Input: part model. Units: mm. Frame: model coordinates. Face numbers are marked on the shaded views. A direction names the side the tool comes from. Coordinates: 2 decimals unless noted, no trailing zeros. Order: outer loops, then holes, each group sorted by start corner. A loop starts at its lowest first (then second) coordinate and runs counter-clockwise, first axis right, second up. Notation, with made-up numbers: (80.5, 39) -> (114.5, 39) arc R14 cw to (114.5, 59) -> close; hole circle Ø5 at (47.25, -27.5). An arc over 180 degrees is marked (long way). Use CSV: the item, a comma, the result in double quotes. Start each with the question number.
```python
from build123d import *

# Parameters (mm, degrees)
SKETCH1_W           = 197.4
SKETCH1_H           = 115
BOSS_EXTRUDE1_DEPTH = 9
BOSS_EXTRUDE2_DEPTH = 10
CUT_EXTRUDE1_DEPTH  = 9
CUT_EXTRUDE2_DEPTH  = 6
CUT_EXTRUDE3_DEPTH  = 2.5


with BuildPart() as part:
    # Sketch1 → Boss-Extrude1 (new body)
    with BuildSketch(Plane.XY):
        with Locations((0, 19.485033023)):
            Rectangle(SKETCH1_W, SKETCH1_H)
    extrude(amount=BOSS_EXTRUDE1_DEPTH)

    # Sketch2 → Boss-Extrude2 (add)
    with BuildSketch(Plane(origin=(0, 76.985033023, 0), x_dir=(1, 0, 0), z_dir=(0, 1, 0))):
        Polygon((-88.7, 10), (88.7, 10), (98.7, 0), (-98.7, 0), align=None)
    extrude(amount=-BOSS_EXTRUDE2_DEPTH)

    # Sketch3 → Cut-Extrude1 (cut)
    with BuildSketch(Plane.XY.offset(9)):
        with BuildLine():
            Line((-80.7, 64.985033023), (-40.7, 64.985033023))
            ThreePointArc((-40.7, 64.985033023), (-36.457359313, 63.22767371), (-34.7, 58.985033023))
            Line((-34.7, 58.985033023), (-34.7, -20.014966977))
            ThreePointArc((-34.7, -20.014966977), (-36.457359313, -24.257607664), (-40.7, -26.014966977))
            Line((-40.7, -26.014966977), (-80.7, -26.014966977))
            ThreePointArc((-80.7, -26.014966977), (-84.942640687, -24.257607664), (-86.7, -20.014966977))
            Line((-86.7, -20.014966977), (-86.7, 58.985033023))
            ThreePointArc((-86.7, 58.985033023), (-84.942640687, 63.22767371), (-80.7, 64.985033023))
        make_face()
    cut_extrude1 = extrude(amount=-CUT_EXTRUDE1_DEPTH, mode=Mode.SUBTRACT)

    # Sketch4 → Cut-Extrude2 (cut)
    with BuildSketch(Plane.XY.offset(9)):
        with BuildLine():
            Line((-94.7, 58.985033023), (-94.7, -20.014966977))
            ThreePointArc((-94.7, -20.014966977), (-90.599494937, -29.914461914), (-80.7, -34.014966977))
            Line((-80.7, -34.014966977), (-40.7, -34.014966977))
            ThreePointArc((-40.7, -34.014966977), (-30.800505063, -29.914461914), (-26.7, -20.014966977))
            Line((-26.7, -20.014966977), (-26.7, 58.985033023))
            ThreePointArc((-26.7, 58.985033023), (-30.800505063, 68.88452796), (-40.7, 72.985033023))
            Line((-40.7, 72.985033023), (-80.7, 72.985033023))
            ThreePointArc((-80.7, 72.985033023), (-90.599494937, 68.88452796), (-94.7, 58.985033023))
        make_face()
    cut_extrude2 = extrude(amount=-CUT_EXTRUDE2_DEPTH, mode=Mode.SUBTRACT)

    # Mirror1: Cut-Extrude1, Cut-Extrude2 across plane
    add(cut_extrude1.mirror(Plane(origin=(0, 0, 0), x_dir=(0, 0, 1), z_dir=(1, 0, 0))), mode=Mode.SUBTRACT)
    add(cut_extrude2.mirror(Plane(origin=(0, 0, 0), x_dir=(0, 0, 1), z_dir=(1, 0, 0))), mode=Mode.SUBTRACT)

    # Sketch5 → Cut-Extrude3 (cut)
    with BuildSketch(Plane(origin=(0, 76.985033023, 0), x_dir=(1, 0, 0), z_dir=(0, 1, 0))):
        with BuildLine():
            Line((-88.7, 5), (88.7, 5))
            ThreePointArc((88.7, 5), (90.613417162, 5.380602337), (92.235533906, 6.464466094))
            Line((92.235533906, 6.464466094), (98.599494937, 0.100505063))
            ThreePointArc((98.599494937, 0.100505063), (94.057568053, -2.934313455), (88.7, -4))
            Line((88.7, -4), (-88.7, -4))
            ThreePointArc((-88.7, -4), (-94.057568053, -2.934313455), (-98.599494937, 0.100505063))
            Line((-98.599494937, 0.100505063), (-92.235533906, 6.464466094))
            ThreePointArc((-92.235533906, 6.464466094), (-90.613417162, 5.380602337), (-88.7, 5))
        make_face()
    extrude(amount=-CUT_EXTRUDE3_DEPTH, mode=Mode.SUBTRACT)


solid = part.part
```
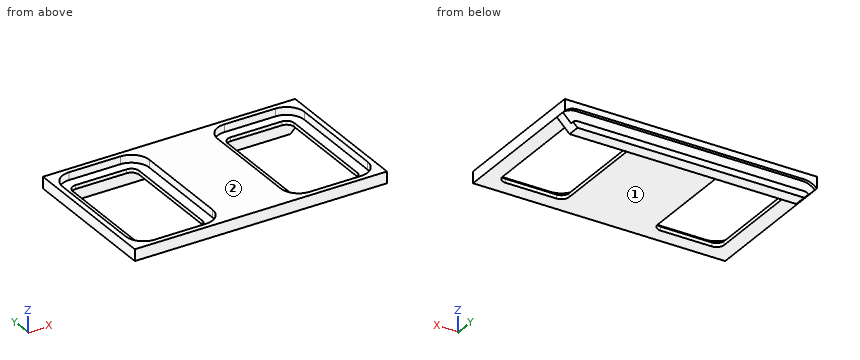
1. Section B-B on y = -9.5. Return loops of the section in (x, z).
2. Material intervals for line 1 along X through (y, z) = (-15.5, 1.25); line 2 along X through (y, z) = (36.5, 5); line 3 along Y through (x, z) = (64.5, 0.75), sorted ascending.
3. Access query for the marked faces 1 and 2. Directions: +Z, -Z, +X, -X, +Y, -Y. A direction counts if a zero-diameter tool reaches every point of the face in a straight line with its end or side. Return the directions, or none.
4. Section A-A on x = 45. Return loops of the section in (y, z), then the cut area to 4 significant figures.
5. Section C-C on z = 6.75. Return loops of the section in (x, y), then the cut area to 3 significant figures.
6. Section D-D on x = -14. Return loops of the section in (y, z), then the cut area to 3 significant figures.
7. Contact query for flat-ended pins moving along their axis: P1, Ø2.5, axis at x = 53.5, z = 2, coming from the +Y side; P2, Ø4, axis at x = -35.5, y = 56.5, coming from the -Z side; P3, Ø1, axis at x = 67.5, z = -5.5, coming from the -Y side. Output: stop coordinate, or through.
Values follow:
1,outline,"(-98.7, 0) -> (-86.7, 0) -> (-86.7, 3) -> (-94.7, 3) -> (-94.7, 9) -> (-98.7, 9) -> close; (-34.7, 0) -> (34.7, 0) -> (34.7, 3) -> (26.7, 3) -> (26.7, 9) -> (-26.7, 9) -> (-26.7, 3) -> (-34.7, 3) -> close; (86.7, 0) -> (98.7, 0) -> (98.7, 9) -> (94.7, 9) -> (94.7, 3) -> (86.7, 3) -> close"
2,line 1,"x = -98.7 to -86.7, -34.7 to 34.7, 86.7 to 98.7"
2,line 2,"x = -98.7 to -94.7, -26.7 to 26.7, 94.7 to 98.7"
2,line 3,"y = -38.01 to -26.01, 64.99 to 74.49"
3,face 1,"-Z, +X, -X, -Y"
3,face 2,"+Z, +X, -X, +Y, -Y"
4,outline,"(-38.01, 0) -> (-26.01, 0) -> (-26.01, 3) -> (-34.01, 3) -> (-34.01, 9) -> (-38.01, 9) -> close; (64.99, 0) -> (66.99, 0) -> (66.99, -10) -> (76.99, -10) -> (76.99, -5) -> (74.49, -5) -> (74.49, 4) -> (76.99, 4) -> (76.99, 9) -> (72.99, 9) -> (72.99, 3) -> (64.99, 3) -> close"
4,area,"197.5 mm2"
5,outline,"(-98.7, -38.01) -> (98.7, -38.01) -> (98.7, 76.99) -> (-98.7, 76.99) -> close; hole (-94.7, -20.01) arc R14 ccw to (-80.7, -34.01) -> (-40.7, -34.01) arc R14 ccw to (-26.7, -20.01) -> (-26.7, 58.99) arc R14 ccw to (-40.7, 72.99) -> (-80.7, 72.99) arc R14 ccw to (-94.7, 58.99) -> close; hole (26.7, -20.01) arc R14 ccw to (40.7, -34.01) -> (80.7, -34.01) arc R14 ccw to (94.7, -20.01) -> (94.7, 58.99) arc R14 ccw to (80.7, 72.99) -> (40.7, 72.99) arc R14 ccw to (26.7, 58.99) -> close"
5,area,"8,490 mm2"
6,outline,"(-38.01, 0) -> (66.99, 0) -> (66.99, -10) -> (76.99, -10) -> (76.99, -5) -> (74.49, -5) -> (74.49, 4) -> (76.99, 4) -> (76.99, 9) -> (-38.01, 9) -> close"
6,area,"1,110 mm2"
7,P1,"stops at y = 74.49"
7,P2,"stops at z = 0"
7,P3,"stops at y = 66.99"
